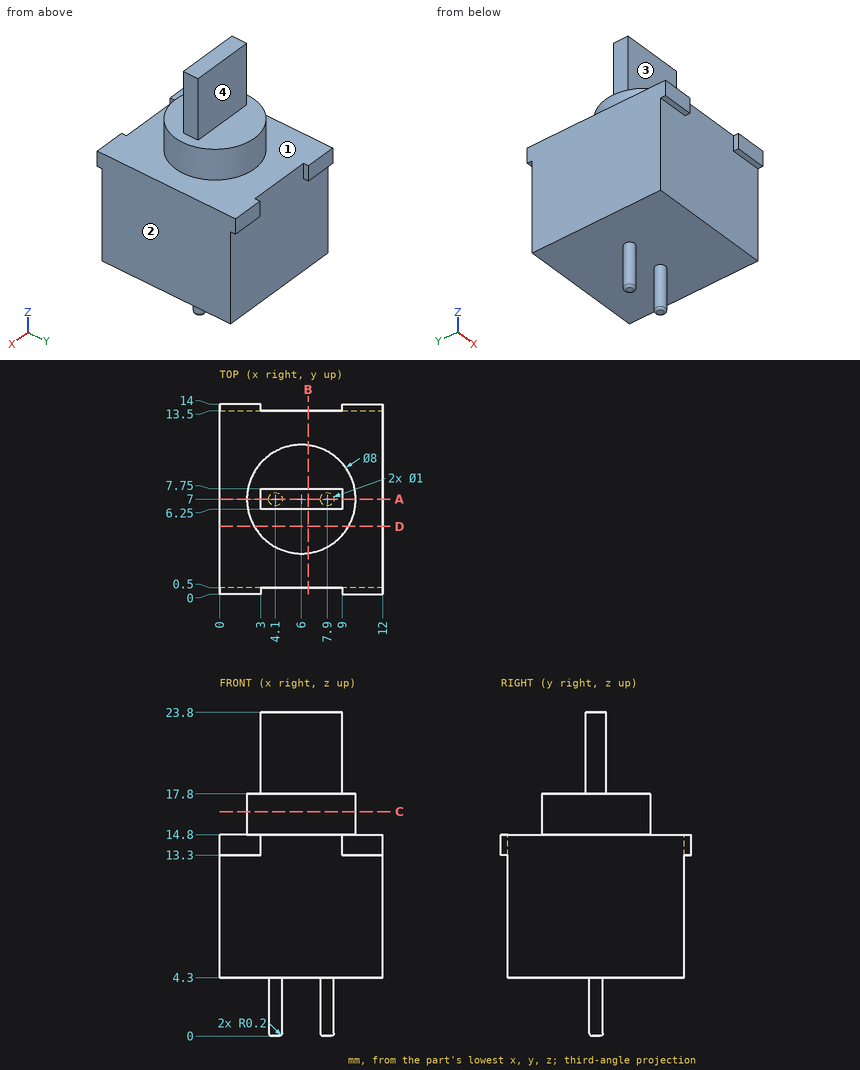
Design review of the part shown in the three views and the two pictorial views. Dimensions are in mm from the part's minimum x, y and z. A direction names the side the tool comes from. Give positions to 0.01 mm unless a question says otherwise; leave off trailing zeros. Write each loop counter-clockwise with the first axis right and the second up, starting at its lowest first coordinate (ties: lowest second). Pieces come first, ordered by that corner, then holes. Notation, with made-up numbers: M 14.25,-33 L 23.25,-33 A38 cw 23.25,6 Z; hole C 88,-26.5 d8. An arc over 180 degrees is marked long. Return JSON: item names as keys, results as strings. Group by question number.
Item 1: Take a section at D-D (y = 5). Give the boundary of the cut face in (x, z), plus the area to 3 significant figures.
Item 2: Take a section at C-C (z = 16.5). Give the boundary of the cut face in (x, y).
Item 3: Wall thickness on line 1 along Z through (x, y) = (7, 12.25); line 2 along Z through (x, y) = (7.5, 9.5); line 3 along Y through (x, z) = (6.5, 6.5): over which ranges is each line inside the solid? List them lowest first.
Item 4: Take a section at B-B (x = 6.5). Give the boundary of the cut face in (y, z).
Item 5: Tool access review of the marked faces 1, 2, 3 and 4: name each direction out of +Z, -Z, +X, -X, +Y, -Y from which nothing blocks a thin tool from reaching the whole face with its end or side.
Item 6: Clearance check with flat-ended pins moving along their axes: pin 1 Ø1 at (x, y) = (7, 5.5) entering from +Z; pin 2 Ø3 at (x, z) = (8, 18.5) entering from -Y; pin 3 Ø3 at (x, z) = (6, 22) entering from -Y. State where each tip first meets the part, or that it passes through.
Item 7: Take a section at A-A (y = 7). Give the boundary of the cut face in (x, z), plus the area to 3 significant figures.
Return value:
{
 "1": {"outline": "M 0,4.3 L 12,4.3 L 12,14.8 L 9.46,14.8 L 9.46,17.8 L 2.54,17.8 L 2.54,14.8 L 0,14.8 Z", "area": "147 mm2"},
 "2": {"outline": "C 6,7 d8"},
 "3": {"line 1": "z = 4.3 to 14.8", "line 2": "z = 4.3 to 17.8", "line 3": "y = 0.5 to 13.5"},
 "4": {"outline": "M 0.5,4.3 L 13.5,4.3 L 13.5,14.8 L 10.97,14.8 L 10.97,17.8 L 7.75,17.8 L 7.75,23.8 L 6.25,23.8 L 6.25,17.8 L 3.03,17.8 L 3.03,14.8 L 0.5,14.8 Z"},
 "5": {"face 1": "+Z", "face 2": "+Z, -Z, +X, +Y, -Y", "face 3": "+Z, +X, -X, -Y", "face 4": "+Z, +X, -X, +Y"},
 "6": {"pin 1": "stops at z = 17.8", "pin 2": "stops at y = 3.06", "pin 3": "stops at y = 6.25"},
 "7": {"outline": "M 0,4.3 L 3.6,4.3 L 3.6,0.2 A0.2 ccw 3.8,0 L 4.4,0 A0.2 ccw 4.6,0.2 L 4.6,4.3 L 7.4,4.3 L 7.4,0.2 A0.2 ccw 7.6,0 L 8.2,0 A0.2 ccw 8.4,0.2 L 8.4,4.3 L 12,4.3 L 12,14.8 L 10,14.8 L 10,17.8 L 9,17.8 L 9,23.8 L 3,23.8 L 3,17.8 L 2,17.8 L 2,14.8 L 0,14.8 Z", "area": "195 mm2"}
}
